Here's how the part is built. I have some questions about the finished solid (model axes, mm). Face numbers are marked on the shaded views. A direction names the side the tool comes from. Round coordinates to 2 decimals unless told otherwise and drop trailing zeros. Write each loop counter-clockwise with the first axis right and the second up, starting at its lowest first coordinate (ties: lowest second). Pieces come first, ordered by that corner, then holes. Notation, with made-up numbers: (42, 50.25) - (51, 50.25) arc R28 ccw to (51, 73.25) - close; hole circle Ø9 at (-36, 67). An arc over 180 degrees is marked (long way). Return JSON: item names as keys, results as strings. Group by question number.
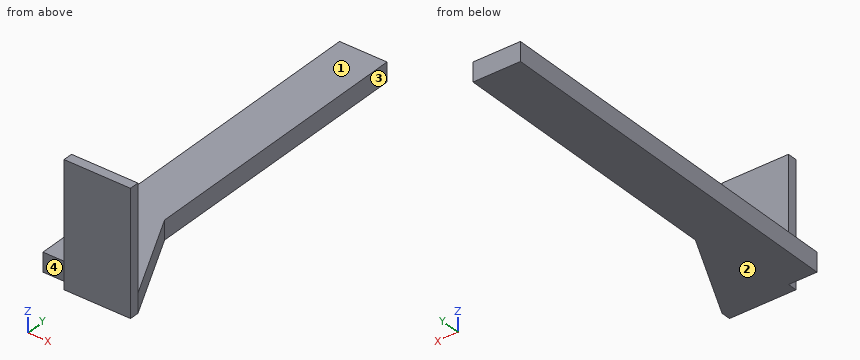
```python
from build123d import *

# Parameters (mm, degrees)
SKETCH1_W           = 35
SKETCH1_H           = 65
BOSS_EXTRUDE1_DEPTH = 5
BOSS_EXTRUDE2_DEPTH = 10


with BuildPart() as part:
    # Sketch1 → Boss-Extrude1 (new body)
    with BuildSketch(Plane(origin=(0, 0, 0), x_dir=(1, 0, 0), z_dir=(0, 1, 0))):
        with Locations((-17.5, -32.5)):
            Rectangle(SKETCH1_W, SKETCH1_H)
    extrude(amount=BOSS_EXTRUDE1_DEPTH)

    # Sketch2 → Boss-Extrude2 (add)
    with BuildSketch(Plane.XY):
        Polygon((0, 5), (-25, 55), (-25, 205), (-50, 205), (-50, 5), align=None)
    extrude(amount=BOSS_EXTRUDE2_DEPTH)


solid = part.part
```
1) Imagine slicing it at C-C (y = 142). Please give me the cut outline in (x, z).
2) I need wall thicknesses on line 1 along Y through (x, z) = (-5.5, 48); line 2 along X through (y, z) = (61.5, 4.5); line 3 along Z through (x, y) = (-25, 53). Which ranges of each line are inside material? Lowest first, please.
3) Imagine slicing it at A-A (x = -19.5). Please give me the cut outline in (y, z).
4) Imagine slicing it at B-B (z = 7). Please give me the cut outline in (x, y).
5) Imagine slicing it at D-D (x = -32.5). Please give me the cut outline in (y, z), plus the area to 4 significant figures.
6) For the marked faces 1, 2, 3 and 4, which set-ups out of +Z, -Z, +X, -X, +Y, -Y let a thin tool reach every point of the face, with its end or its side?
7) Will these pins go through, and if not, where does the flat tip stop? pin 1 Ø8 at (x, z) = (-39.5, 4.5) entering from -Y; pin 2 Ø5 at (y, z) = (123, 4.5) entering from +X; pin 3 Ø10.5 at (x, z) = (-18, 38.5) entering from +Y.
Results found:
{
 "1": {"outline": "(-50, 0) - (-25, 0) - (-25, 10) - (-50, 10) - close"},
 "2": {"line 1": "y = 0 to 5", "line 2": "x = -50 to -25", "line 3": "z = 0 to 10"},
 "3": {"outline": "(0, 0) - (44, 0) - (44, 10) - (5, 10) - (5, 65) - (0, 65) - close"},
 "4": {"outline": "(-50, 5) - (-35, 5) - (-35, 0) - (0, 0) - (0, 5) - (-25, 55) - (-25, 205) - (-50, 205) - close"},
 "5": {"outline": "(0, 0) - (205, 0) - (205, 10) - (5, 10) - (5, 65) - (0, 65) - close", "area": "2,325 mm²"},
 "6": {"face 1": "+Z, +X, -X, +Y", "face 2": "-Z, +X, -X, +Y, -Y", "face 3": "+Z, -Z, +X, +Y", "face 4": "+Z, -Z, -X, -Y"},
 "7": {"pin 1": "stops at y = 5", "pin 2": "stops at x = -25", "pin 3": "stops at y = 5"}
}
